```python
from build123d import *

# Parameters (mm, degrees)
SKETCH1_R               = 24
SKETCH1_R_2             = 14
BOSS_EXTRUDE1_DEPTH     = 50.5
SKETCH5_R               = 14
SKETCH5_R_2             = 6.75
BOSS_EXTRUDE3_DEPTH     = 6
FILLET3_R               = 4
FILLET1_R               = 10
FILLET2_R               = 10
SKETCH2_R               = 4.5
CUT_EXTRUDE1_DEPTH      = 50.5
CUT_EXTRUDE1_DEPTH_BACK = 50.5
SKETCH4_W               = 80
SKETCH4_H               = 50.5
SKETCH4_R               = 2.05
BOSS_EXTRUDE2_DEPTH     = 5


with BuildPart() as part:
    # Sketch1 → Boss-Extrude1 (new body)
    with BuildSketch(Plane.XY):
        Circle(SKETCH1_R)
        Circle(SKETCH1_R_2, mode=Mode.SUBTRACT)
        with BuildLine():
            Line((-40, 0), (-40, -24.5))
            Line((-40, -24.5), (40, -24.5))
            Line((40, -24.5), (40, 0))
            Line((40, 0), (24, 0))
            ThreePointArc((24, 0), (0, -24), (-24, 0))
            Line((-24, 0), (-40, 0))
        make_face()
    extrude(amount=BOSS_EXTRUDE1_DEPTH)

    # Sketch5 → Boss-Extrude3 (add)
    with BuildSketch(Plane.XY.offset(50.5)):
        Circle(SKETCH5_R)
        Circle(SKETCH5_R_2, mode=Mode.SUBTRACT)
    extrude(amount=-BOSS_EXTRUDE3_DEPTH)

    # Fillet3
    fillet3_edges = [part.edges().sort_by_distance(p)[0] for p in [
        (-14, 0, 44.5),
    ]]
    fillet(fillet3_edges, radius=FILLET3_R)

    # Fillet1
    fillet1_edges = [part.edges().sort_by_distance(p)[0] for p in [
        (40, 0, 25.25),
        (-40, 0, 25.25),
    ]]
    fillet(fillet1_edges, radius=FILLET1_R)

    # Fillet2
    fillet2_edges = [part.edges().sort_by_distance(p)[0] for p in [
        (-24, 0, 25.25),
        (24, 0, 25.25),
    ]]
    fillet(fillet2_edges, radius=FILLET2_R)

    # Sketch2 → Cut-Extrude1 (cut, two sides)
    with BuildSketch(Plane(origin=(0, 0, 0), x_dir=(1, 0, 0), z_dir=(0, 1, 0))) as cut_extrude1_sk:
        with Locations(Location((28.5, -25.25, 0), (0, 0, 51.961063879))):
            Circle(SKETCH2_R)
        with Locations(Location((-28.5, -25.25, 0), (0, 0, 128.038935344))):
            Circle(SKETCH2_R)
    extrude(amount=CUT_EXTRUDE1_DEPTH, mode=Mode.SUBTRACT)
    extrude(cut_extrude1_sk.sketch, amount=-CUT_EXTRUDE1_DEPTH_BACK, mode=Mode.SUBTRACT)

    # Sketch4 → Boss-Extrude2 (add)
    with BuildSketch(Plane.XZ.offset(24.5)):
        with Locations((0, 25.25)):
            Rectangle(SKETCH4_W, SKETCH4_H)
        with Locations(Location((-28.5, 25.25, 0), (0, 0, 270))):
            Circle(SKETCH4_R, mode=Mode.SUBTRACT)
        with Locations(Location((28.5, 25.25, 0), (0, 0, 270))):
            Circle(SKETCH4_R, mode=Mode.SUBTRACT)
    extrude(amount=-BOSS_EXTRUDE2_DEPTH)


solid = part.part
```
CAD build for the part. Positions are in the model's coordinates, mm. A direction names the side the tool comes from. Give positions to 0.01 mm unless a question says otherwise; leave off trailing zeros. Write each loop counter-clockwise with the first axis right and the second up, starting at its lowest first coordinate (ties: lowest second). Pieces come first, ordered by that corner, then holes. Notation, with made-up numbers: (78, -11) -> (128, -11) arc R24 cw to (128, 0) -> close; hole circle Ø2 at (43.5, 36). An arc over 180 degrees is marked (long way). Write each question's results on one line, items separated by ' | '.
1. Wall check: probe 1 along Y at (x, z) = (0, 46.9); probe 2 along Y at (x, z) = (0, 24); probe 3 along X at (y, z) = (-8, 23.5). Give the ranges that are in metal, low to high. Write a range as [from, to].
Geometry check:
probe 1: [-24.5, -6.75], [6.75, 24] | probe 2: [-24.5, -14], [14, 24] | probe 3: [-39.8, -32.65], [-24.35, -11.49], [11.49, 24.35], [32.65, 39.8]
2. Two-plate mould, pull along Z, no slides. Class faces 4 (the cylindrical face through (12.932, -5.362, 19.966)), 5 (the flat face through (-9, -11, 0)), 6 (the flat face through (-28, -19.5, 23)), 7 (the flat face through (-1, -11, 50.5)): pulls with the +Z half, pulls with the -Z half, needs draft (parallel to the pull), parting line crosses it, or undercut.
Geometry check:
face 4: needs draft | face 5: pulls with the -Z half | face 6: undercut | face 7: pulls with the +Z half
3. Drop flat-ended pins along their axis: P1, Ø1.5, axis at y = 3.5, z = 29, coming from the -X side; P2, Ø3, axis at x = -1, y = 9.5, coming from the -Z side; P3, Ø1.5, axis at y = 7.5, z = 21.5, coming from the +X side. Give the stop position or say it passes through.
Geometry check:
P1: x = -25.49 | P2: z = 44.36 | P3: x = 23.03
4. Cut at D-D, the plane y = 15.5. Write the cut outline in (x, z), then the cut area to 3 significant figures.
Geometry check:
outline: (-18.32, 0) -> (18.32, 0) -> (18.32, 50.5) -> (-18.32, 50.5) -> close | area: 1,850 mm²
5. Cut at A-A, the plane y = -2.5. Give the number of separate pieces and of enclosed holes in the cut face, then the cut area to 3 significant figures.
Geometry check:
separate pieces: 2 | enclosed holes: 2 | area: 2,280 mm²
6. Which spindle directions (+Z, -Z, +X, -X, +Y, -Y) get a long thin tool onto all of the face, cutting with end or side? Do faces 1 (the flat face through (29, -19.5, 23)), 2 (the flat face through (7, -2, 44.5)), 3 (the cylindrical face through (30.533, -22.035, 25.517)). Say none if no direction does.
Geometry check:
face 1: +Y | face 2: -Z | face 3: +Y, -Y
7. Cut at C-C, the plane x = -16. Write the cut outline in (y, z), then the cut area to 3 significant figures.
Geometry check:
outline: (-24.5, 0) -> (17.89, 0) -> (17.89, 50.5) -> (-24.5, 50.5) -> close | area: 2,140 mm²
